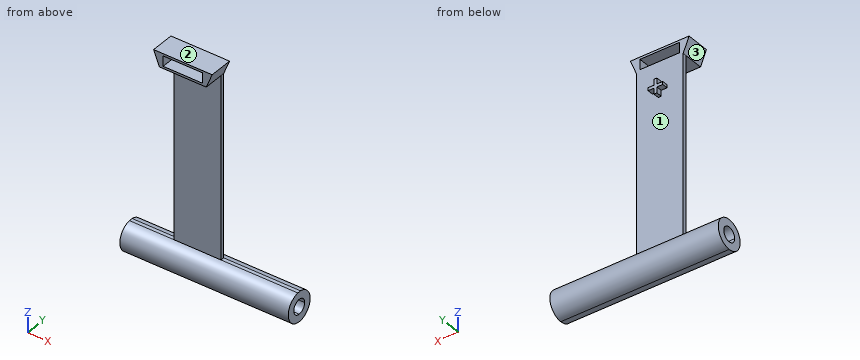
```python
from build123d import *

# Parameters (mm, degrees)
BOSS_EXTRUDE2_DEPTH      = 32
SKETCH5_W                = 54
SKETCH5_H                = 14
CUT_EXTRUDE1_DEPTH       = 32
SKETCH6_W                = 64
SKETCH6_H                = 5
BOSS_EXTRUDE3_DEPTH      = 70
SKETCH7_W                = 2
SKETCH7_H                = 8
SKETCH7_H_2              = 2
SKETCH7_W_2              = 8
BOSS_EXTRUDE4_DEPTH      = 8
SKETCH8_W                = 64
SKETCH8_H                = 5
BOSS_EXTRUDE5_DEPTH      = 178
BOSS_EXTRUDE7_DEPTH      = 105
BOSS_EXTRUDE7_DEPTH_BACK = 125
CUT_EXTRUDE4_DEPTH       = 264


with BuildPart() as part:
    # Sketch4 → Boss-Extrude2 (new body)
    with BuildSketch(Plane(origin=(0, 0, 0), x_dir=(1, 0, 0), z_dir=(0, 1, 0))):
        Polygon((8, 20), (0, 0), (80, 0), (72, 20), align=None)
    extrude(amount=BOSS_EXTRUDE2_DEPTH)

    # Sketch5 → Cut-Extrude1 (cut)
    with BuildSketch(Plane(origin=(0, 32, 0), x_dir=(1, 0, 0), z_dir=(0, 1, 0))):
        with Locations((40, 10)):
            Rectangle(SKETCH5_W, SKETCH5_H)
    extrude(amount=-CUT_EXTRUDE1_DEPTH, mode=Mode.SUBTRACT)

    # Sketch6 → Boss-Extrude3 (add)
    with BuildSketch(Plane(origin=(0, 0, -20), x_dir=(-1, 0, 0), z_dir=(0, 0, -1))):
        with Locations((-40, 29.5)):
            Rectangle(SKETCH6_W, SKETCH6_H)
    extrude(amount=BOSS_EXTRUDE3_DEPTH)

    # Sketch7 → Boss-Extrude4 (add)
    with BuildSketch(Plane(origin=(0, 32, 0), x_dir=(1, 0, 0), z_dir=(0, 1, 0))):
        with Locations((41, 61)):
            Rectangle(SKETCH7_W, SKETCH7_H)
        with Locations((39, 61)):
            Rectangle(SKETCH7_W, SKETCH7_H)
        with Locations((39, 56)):
            Rectangle(SKETCH7_W, SKETCH7_H_2)
        with Locations((41, 56)):
            Rectangle(SKETCH7_W, SKETCH7_H_2)
        with Locations((34, 56)):
            Rectangle(SKETCH7_W_2, SKETCH7_H_2)
        with Locations((34, 54)):
            Rectangle(SKETCH7_W_2, SKETCH7_H_2)
        with Locations((39, 54)):
            Rectangle(SKETCH7_W, SKETCH7_H_2)
        with Locations((41, 54)):
            Rectangle(SKETCH7_W, SKETCH7_H_2)
        with Locations((41, 49)):
            Rectangle(SKETCH7_W, SKETCH7_H)
        with Locations((39, 49)):
            Rectangle(SKETCH7_W, SKETCH7_H)
        with Locations((46, 54)):
            Rectangle(SKETCH7_W_2, SKETCH7_H_2)
        with Locations((46, 56)):
            Rectangle(SKETCH7_W_2, SKETCH7_H_2)
    extrude(amount=BOSS_EXTRUDE4_DEPTH)

    # Sketch8 → Boss-Extrude5 (add)
    with BuildSketch(Plane(origin=(0, 0, -90), x_dir=(-1, 0, 0), z_dir=(0, 0, -1))):
        with Locations((-40, 29.5)):
            Rectangle(SKETCH8_W, SKETCH8_H)
    extrude(amount=BOSS_EXTRUDE5_DEPTH)

    # Sketch13 → Boss-Extrude7 (add, two sides: drawn at the far end of the back side and taken through both)
    with BuildSketch(Plane(origin=(72, 0, 0), x_dir=(0, 0, -1), z_dir=(1, 0, 0)).offset(-BOSS_EXTRUDE7_DEPTH_BACK)):
        with BuildLine():
            ThreePointArc((268, 27), (289.252420174, 9.383304354), (308.155644371, 29.5))
            ThreePointArc((308.155644371, 29.5), (289.252420174, 49.616695646), (268, 32))
            Line((268, 32), (268, 29.5))
            Line((268, 29.5), (268, 27))
        make_face()
    extrude(amount=BOSS_EXTRUDE7_DEPTH + BOSS_EXTRUDE7_DEPTH_BACK)

    # Sketch14 → Cut-Extrude4 (cut)
    with BuildSketch(Plane(origin=(177, 0, 0), x_dir=(0, 0, -1), z_dir=(1, 0, 0))):
        with BuildLine():
            ThreePointArc((298, 29.5), (295.071067812, 36.571067812), (288, 39.5))
            Line((288, 39.5), (288, 19.5))
            ThreePointArc((288, 19.5), (295.071067812, 22.428932188), (298, 29.5))
        make_face()
        with BuildLine():
            Line((288, 19.5), (288, 39.5))
            ThreePointArc((288, 39.5), (278, 29.5), (288, 19.5))
        make_face()
    extrude(amount=-CUT_EXTRUDE4_DEPTH, mode=Mode.SUBTRACT)


solid = part.part
```
The model under review builds one solid part; all positions refer to its coordinate system, in mm. Face numbers are marked on the shaded views. Round coordinates to 2 decimals unless told otherwise and drop trailing zeros. Write each loop counter-clockwise with the first axis right and the second up, starting at its lowest first coordinate (ties: lowest second). Pieces come first, ordered by that corner, then holes. Notation, with made-up numbers: (-6, -8.5) - (13, -8.5) arc R21 ccw to (13, 27.5) - close; hole circle Ø11 at (50, 53.5). An arc over 180 degrees is marked (long way). One line per question, with ' | ' between items.
Item 1: The part is to be moulded in two halves that separate along Z. For the marked faces 1, 2 and 3, say which applies: pulls with the +Z half, pulls with the -Z half, needs draft (parallel to the pull), parting line crosses it, or undercut.
Resolved:
face 1: undercut | face 2: pulls with the +Z half | face 3: undercut
Item 2: Add section B-B, the plane x = -28. Give the boundary of the cut face in (y, z).
Resolved:
outline: (27, -268) arc R20.16 ccw (long way) to (32, -268) - close; hole circle Ø20 at (29.5, -288)
Item 3: For P1, Ø2.5, axis at y = 37, z = -60, coming from the +X side; P2, Ø6, axis at y = 42, z = -70.5, coming from the +X side (1 decimal); P3, Ø2.5, axis at x = 46.5, y = 37.5, coming from the +Z side; P4, Ø9, axis at x = 35, y = 37, coming from the -Z side, all flat-tipped, find the tip position at first contact; note any pin that passes through.
Resolved:
P1: stops at x = 42 | P2: passes through | P3: stops at z = -53 | P4: stops at z = -307.93
Item 4: Add section A-A, the plane x = 34.5. Give the boundary of the cut face in (y, z).
Resolved:
outline: (0, -20) - (27, -20) - (27, -268) arc R20.16 ccw (long way) to (32, -268) - (32, -57) - (40, -57) - (40, -53) - (32, -53) - (32, -17) - (0, -17) - close; (0, -3) - (32, -3) - (32, 0) - (0, 0) - close; hole circle Ø20 at (29.5, -288)
Item 5: To check wall thickness, follow probe 1 along Z at (x, y) = (-6.5, 36); probe 2 along Z at (x, y) = (-29.5, 38); probe 3 along Z at (x, y) = (-39, 12). State the ranges of each line that lie inside material, in increasing order.
Resolved:
probe 1: z = -307.08 to -295.6, -280.4 to -268.92 | probe 2: z = -306.28 to -293.27, -282.73 to -269.72 | probe 3: z = -298 to -278
Item 6: Add section C-C, the plane y = 46. Give the boundary of the cut face in (x, z), then the cut area to 3 significant figures.
Resolved:
outline: (-53, -299.58) - (177, -299.58) - (177, -276.42) - (-53, -276.42) - close | area: 5,320 mm2
